```python
from build123d import *

# Parameters (mm, degrees)
F1_DEPTH = 15
F2_SIZE2 = 3
F2_SIZE  = 13
F3_SIZE2 = 3
F3_SIZE  = 13
F4_R     = 3
F5_DEPTH = 25
F6_W     = 2
F6_H     = 0.5
F6_H_2   = 2
F7_DEPTH = 1
F8_W     = 2
F8_H     = 0.5
F8_H_2   = 2
F9_DEPTH = 1


with BuildPart() as f1:
    # F0 (on Top) → F1 (new body)
    with BuildSketch(Plane.XY):
        with BuildLine():
            Line((-17.5, 2.5), (-15.0505102572, 2.5))
            ThreePointArc((-15.0505102572, 2.5), (-17.5, 3.5), (-19.9494897428, 2.5))
            Line((-19.9494897428, 2.5), (-17.5, 2.5))
        make_face()
        with BuildLine():
            ThreePointArc((-17.5, -2.5), (-20, 0), (-17.5, 2.5))
            Line((-17.5, 2.5), (-19.9494897428, 2.5))
            ThreePointArc((-19.9494897428, 2.5), (-20.7267021942, 1.3558735008), (-21, 0))
            ThreePointArc((-21, 0), (-20.7267021942, -1.3558735008), (-19.9494897428, -2.5))
            Line((-19.9494897428, -2.5), (-17.5, -2.5))
        make_face()
        with BuildLine():
            ThreePointArc((-19.9494897428, -2.5), (-17.5, -3.5), (-15.0505102572, -2.5))
            Line((-15.0505102572, -2.5), (-17.5, -2.5))
            Line((-17.5, -2.5), (-19.9494897428, -2.5))
        make_face()
        with BuildLine():
            ThreePointArc((-14, 0), (-14.2732978058, 1.3558735008), (-15.0505102572, 2.5))
            Line((-15.0505102572, 2.5), (-17.5, 2.5))
            ThreePointArc((-17.5, 2.5), (-15.732233047, 1.767766953), (-15, 0))
            ThreePointArc((-15, 0), (-15.732233047, -1.767766953), (-17.5, -2.5))
            Line((-17.5, -2.5), (-15.0505102572, -2.5))
            ThreePointArc((-15.0505102572, -2.5), (-14.2732978058, -1.3558735008), (-14, 0))
        make_face()
        with BuildLine():
            ThreePointArc((15.0505102572, -2.5), (14, 0), (15.0505102572, 2.5))
            Line((15.0505102572, 2.5), (-15.0505102572, 2.5))
            ThreePointArc((-15.0505102572, 2.5), (-14.2732978058, 1.3558735008), (-14, 0))
            ThreePointArc((-14, 0), (-14.2732978058, -1.3558735008), (-15.0505102572, -2.5))
            Line((-15.0505102572, -2.5), (15.0505102572, -2.5))
        make_face()
        with BuildLine():
            ThreePointArc((17.5, -2.5), (15, 0), (17.5, 2.5))
            Line((17.5, 2.5), (15.0505102572, 2.5))
            ThreePointArc((15.0505102572, 2.5), (14, 0), (15.0505102572, -2.5))
            Line((15.0505102572, -2.5), (17.5, -2.5))
        make_face()
        with BuildLine():
            Line((17.5, 2.5), (19.9494897428, 2.5))
            ThreePointArc((19.9494897428, 2.5), (17.5, 3.5), (15.0505102572, 2.5))
            Line((15.0505102572, 2.5), (17.5, 2.5))
        make_face()
        with BuildLine():
            ThreePointArc((21, 0), (20.7267021942, 1.3558735008), (19.9494897428, 2.5))
            Line((19.9494897428, 2.5), (17.5, 2.5))
            ThreePointArc((17.5, 2.5), (19.267766953, 1.767766953), (20, 0))
            ThreePointArc((20, 0), (19.267766953, -1.767766953), (17.5, -2.5))
            Line((17.5, -2.5), (19.9494897428, -2.5))
            ThreePointArc((19.9494897428, -2.5), (20.7267021942, -1.3558735008), (21, 0))
        make_face()
        with BuildLine():
            ThreePointArc((15.0505102572, -2.5), (17.5, -3.5), (19.9494897428, -2.5))
            Line((19.9494897428, -2.5), (17.5, -2.5))
            Line((17.5, -2.5), (15.0505102572, -2.5))
        make_face()
    extrude(amount=F1_DEPTH)

    # F2
    f2_edges = [f1.edges().sort_by_distance(p)[0] for p in [
        (0, -2.5, 15),
    ]]
    f2_side = f1.faces().sort_by_distance((0, -2.5, 7.5))[0]
    chamfer(f2_edges, length=F2_SIZE, length2=F2_SIZE2, reference=f2_side)

    # F3
    f3_edges = [f1.edges().sort_by_distance(p)[0] for p in [
        (0, 2.5, 0),
    ]]
    f3_side = f1.faces().sort_by_distance((0, 2.5, 7.5))[0]
    chamfer(f3_edges, length=F3_SIZE, length2=F3_SIZE2, reference=f3_side)

    # F4 (on face) → F5 (cut)
    with BuildSketch(Plane(origin=(0, -0.4747191011, 0.1095505618), x_dir=(-1, 0, 0), z_dir=(0, 0.9743911957, -0.2248595067))):
        with Locations((0, 6.6146171554)):
            Circle(F4_R)
    extrude(amount=-F5_DEPTH, mode=Mode.SUBTRACT)

    # F6 (on face) → F7 (cut)
    with BuildSketch(Plane.XY.offset(15)):
        with Locations((7, 0.25)):
            Rectangle(F6_W, F6_H)
        with Locations((-7, 0.25)):
            Rectangle(F6_W, F6_H)
        with Locations((-7, 1.5)):
            Rectangle(F6_W, F6_H_2)
        with Locations((-7, 2.75)):
            Rectangle(F6_W, F6_H)
        with Locations((7, 1.5)):
            Rectangle(F6_W, F6_H_2)
        with Locations((7, 2.75)):
            Rectangle(F6_W, F6_H)
    extrude(amount=-F7_DEPTH, mode=Mode.SUBTRACT)

    # F8 (on face) → F9 (cut)
    with BuildSketch(Plane(origin=(0, 0, 0), x_dir=(1, 0, 0), z_dir=(0, 0, -1))):
        with Locations((7, 0.25)):
            Rectangle(F8_W, F8_H)
        with Locations((7, 1.5)):
            Rectangle(F8_W, F8_H_2)
        with Locations((7, 2.75)):
            Rectangle(F8_W, F8_H)
        with Locations((-7, 0.25)):
            Rectangle(F8_W, F8_H)
        with Locations((-7, 1.5)):
            Rectangle(F8_W, F8_H_2)
        with Locations((-7, 2.75)):
            Rectangle(F8_W, F8_H)
    extrude(amount=-F9_DEPTH, mode=Mode.SUBTRACT)


solid = f1.part
```
The model under review builds one solid part; all positions refer to its coordinate system, in mm. A direction names the side the tool comes from. Coordinates: 2 decimals unless noted, no trailing zeros. Write each loop counter-clockwise with the first axis right and the second up, starting at its lowest first coordinate (ties: lowest second). Pieces come first, ordered by that corner, then holes.
1) The part is to be moulded in two halves that separate along X. For faces 1 (the face through (-7, 1, 14)), 2 (the face through (0, 2, 15)), say which applies: pulls with the +X half, pulls with the -X half, needs draft (parallel to the pull), parting line crosses it, or undercut.
2) Clearance check with flat-ended pins moving along their axes: pin 1 Ø0.8 at (y, z) = (-1, 0.5) entering from -X; pin 2 Ø1 at (y, z) = (-1.5, 11) entering from +X; pin 3 Ø8 at (x, z) = (-0.5, 4) entering from -Y. State where each tip first meets the part, or that it passes through.
3) Machinability: for faces 3 (the face through (-8, -1.4, 0.5)), 4 (the face through (0, -2.5, 1)), 5 (the face through (8, 1.4, 14.5)), which of the approach directions +Z, -Z, +X, -X, +Y, -Y give a long, thin tool a straight path to every point of the face, cutting with its end or side? Answer none if there is none.
4) We need section B-B on z = 13.5. State the section outline as (x, y) points.
5) To check wall thickness, follow probe 1 along X at (y, z) = (-2.25, 8.75); probe 2 along X at (y, z) = (1.5, 1.25); probe 3 along Y at (x, z) = (18.5, 2). State the ranges of each line that lie inside material, in increasing order.
6) We need section D-D on z = 7.5. Count the separate pieces of the cut face and the enclosed holes in it, then the cut area to 3 significant figures.
7) We need section A-A on x = 2.5. State the section outline as (y, z) points, then the cut area to 3 significant figures.
8) We need section C-C on x = 12. State the section outline as (y, z) points, then the cut area to 3 significant figures.
Answer list:
1. face 1: undercut
1. face 2: needs draft
2. pin 1: stops at x = -20.95
2. pin 2: stops at x = 20.85
2. pin 3: stops at y = -2.5
3. face 3: -Z, +Y, -Y
3. face 4: +Z, -Z, -Y
3. face 5: +Z, +Y, -Y
4. outline: (-15.05, 2.5) arc R3.5 ccw (long way) to (-14, 0.15) - (14, 0.15) arc R3.5 ccw (long way) to (15.05, 2.5) - close; hole circle Ø5 at (-17.5, 0); hole circle Ø5 at (17.5, 0)
5. probe 1: x = -20.18 to -18.59, -16.41 to -14.82, 14.82 to 16.41, 18.59 to 20.18
5. probe 2: x = -20.66 to -19.5, -15.5 to -14.34, 14.34 to 15.5, 19.5 to 20.66
5. probe 3: y = -3.35 to -2.29, 2.29 to 3.35
6. separate pieces: 2
6. enclosed holes: 2
6. area: 92.6 mm2
7. outline: (-2.5, 0) - (-0.5, 0) - (0.64, 4.94) - (-1.7, 5.48) - (-2.5, 2) - close; (-0.95, 8.71) - (1.39, 8.17) - (2.5, 13) - (2.5, 15) - (0.5, 15) - close
7. area: 28.0 mm2
8. outline: (-2.5, 0) - (-0.5, 0) - (2.5, 13) - (2.5, 15) - (0.5, 15) - (-2.5, 2) - close
8. area: 36.0 mm2
